Autodesk Inventor part; units mm, degrees
ref_plane "YZ Plane" through (0, 0, 0) normal (1, 0, 0) x (0, 1, 0)
ref_plane "XZ Plane" through (0, 0, 0) normal (0, 1, 0) x (-1, 0, 0)
ref_plane "XY Plane" through (0, 0, 0) normal (0, 0, 1) x (1, 0, 0)
sketch "Sketch1" plane through (0, 0, 0) normal (0, 0, 1) x (1, 0, 0)
  line L0 (-37, 85) -> (37, 85)
  line L1 (37, 85) -> (37, -85)
  line L2 (37, -85) -> (-37, -85)
  line L3 (-37, -85) -> (-37, 85)
  line L4 (-37, 85) -> (37, -85) construction
  line L5 (37, 85) -> (-37, -85) construction
  line L6 (22, 85) -> (-22, 85)
  line L7 (-22, 85) -> (-22, 62)
  line L8 (-22, 62) -> (22, 62)
  line L9 (22, 62) -> (22, 85)
  point P0 (0, 0)
  point P1 (0, 62)
  point P2 (0, 85)
  point P3 (-22, 85)
  dimension "d0" = 74
  dimension "d1" = 170
  dimension "d9" = 44
  dimension "d10" = 23
extrude "Extrusion1" add sketch "Sketch1" along normal blind 5 contours L0 L7 L8 L9 L1 L2 L3
sketch "Sketch2" plane through (0, 0, 0) normal (0, 0, -1) x (-1, 0, 0)
  circle A0 centre (-26, 81) radius 2.5
  line L0 (0, 0) -> (0, 85)
  line L1 (-37, 85) -> (37, 85)
  circle A1 centre (26, 81) radius 2.5
  dimension "d4" = 5
  dimension "d5" = 52
  dimension "d8" = 4
extrude "Extrusion2" cut sketch "Sketch2" against normal blind 4
sketch "Sketch3" plane through (0, 0, 0) normal (0, 0, -1) x (-1, 0, 0)
  line L0 (37, -85) -> (-37, -85)
  line L1 (-37, 85) -> (-37, -85)
  line L2 (-37, -85) -> (37, -85)
  line L3 (37, -85) -> (37, 85)
  line L4 (33, 85) -> (33, -81)
  line L5 (33, -81) -> (-33, -81)
  line L6 (-33, -81) -> (-33, 85)
  line L7 (-37, 85) -> (-22, 85)
  line L8 (-37, 85) -> (-33, 85)
  line L9 (22, 85) -> (37, 85)
  line L10 (33, 85) -> (37, 85)
  line L11 (-33, -81) -> (-27.5, -81)
  line L12 (-27.5, -81) -> (-27.5, -28.7771)
  line L13 (-27.5, -28.7771) -> (-33, -28.7771)
  line L14 (-33, -28.7771) -> (-33, -81)
  line L15 (33, -81) -> (27.5, -81)
  line L16 (27.5, -81) -> (27.5, -28.7771)
  line L17 (27.5, -28.7771) -> (33, -28.7771)
  line L18 (33, -28.7771) -> (33, -81)
  point P0 (0, 0)
  point P1 (33, -28.7771)
  point P2 (-33, -28.7771)
  dimension "d12" = 4
  dimension "d18" = 52.2229
  dimension "d19" = 5.5
  dimension "d20" = 5.5
extrude "Extrusion3" add sketch "Sketch3" along normal blind 22.8316
sketch "Sketch4" plane through (-37, -85, 5) normal (0, -1, 0) x (1, 0, 0)
  line L0 (70, -27.8316) -> (74, -27.8316)
  line L1 (74, -27.8316) -> (0, -27.8316)
  line L2 (0, -27.8316) -> (0, -21.8316)
  line L3 (0, -21.8316) -> (74, -21.8316)
  line L4 (74, -21.8316) -> (74, -27.8316)
  point P0 (37, -5)
  dimension "d15" = 6
  dimension "d21" = 74
extrude "Extrusion4" add sketch "Sketch4" along normal blind 54
chamfer "Chamfer1" distance 10 angle 45 2 edges at (30.25, -28.7771, -22.8316) (-30.25, -28.7771, -22.8316)
sketch "Sketch5" plane through (0, 0, -22.8316) normal (0, 0, -1) x (-1, 0, 0)
  line L0 (-31.85, -29.2771) -> (-31.85, -139.7771)
  line L1 (-31.85, -29.2771) -> (78.65, -29.2771) construction
  circle A0 centre (-31.85, -44.2771) radius 2.5
  circle A1 centre (-31.85, -64.2771) radius 2.5
  circle A2 centre (-31.85, -84.2771) radius 2.5
  circle A3 centre (-31.85, -104.2771) radius 2.5
  circle A4 centre (-31.85, -124.2771) radius 2.5
  line L2 (-27.5, -28.7771) -> (-27.5, -81)
  line L3 (-37, -85) -> (-37, 85)
  line L4 (-27.5, -28.7771) -> (-33, -28.7771)
  line L5 (-37, -139) -> (37, -139)
  line L6 (0, -139) -> (0, -29.2771)
  circle A5 centre (31.85, -44.2771) radius 2.5
  circle A6 centre (31.85, -64.2771) radius 2.5
  circle A7 centre (31.85, -84.2771) radius 2.5
  circle A8 centre (31.85, -104.2771) radius 2.5
  circle A9 centre (31.85, -124.2771) radius 2.5
  point P0 (0, 0)
  point P1 (-31.85, -36)
  dimension "d23" = 110.5
  dimension "d24" = 90
  dimension "d25" = 5
  dimension "d26" = 15
  dimension "d29" = 20
  dimension "d39" = 5.15
  dimension "d40" = 0.5
extrude "Extrusion5" cut sketch "Sketch5" against normal blind 5
fillet "Fillet1" radius 5 4 edges at (37, 0, 5) (-37, 0, 5) (37, -112, -16.8316) (-37, -112, -16.8316)
properties part number "cover^3"
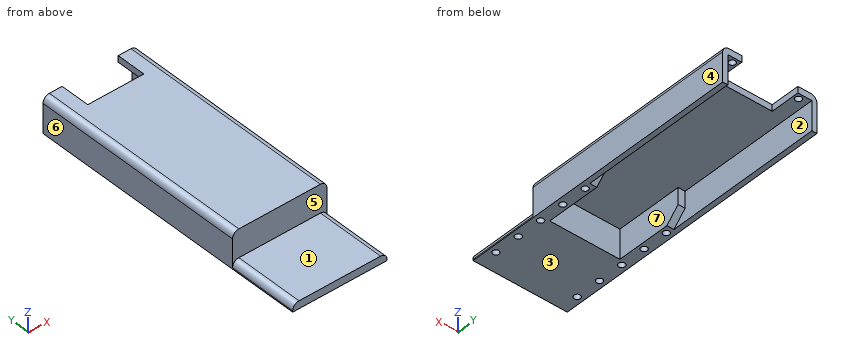
Part model, mm, in its own coordinate system. Face numbers are marked on the shaded views. A direction names the side the tool comes from. Round coordinates to 2 decimals unless told otherwise and drop trailing zeros. Write each loop counter-clockwise with the first axis right and the second up, starting at its lowest first coordinate (ties: lowest second). Pieces come first, ordered by that corner, then holes. Notation, with made-up numbers: (37.25, 44.25) -> (61.25, 44.25) arc R20 ccw to (61.25, 83.25) -> close; hole circle Ø3 at (22.5, -27). An arc over 180 degrees is marked (long way). Return JSON: item names as keys, results as strings. Group by question number.
Q1. Probe L1, parallel to X at y = 70, z = -12.5; L2, parallel to Y at x = 31.85, z = -20.05; L3, parallel to Y at x = 31.85, z = -21.3. List the from-to ranges inside material, lowest first. Write a range as [from, to].
Q2. Pin check, flat tips, straight feed: pin 1 (10 mm diameter, centred on x = -10, y = 2, fed in from -Z); pin 2 (6 mm diameter, centred on x = -10.5, z = -1, fed in from -Y); pin 3 (11.5 mm diameter, centred on x = 9, z = -7.5, fed in from +Y). Stop position of each tip, or through.
Q3. Mould opens along X. For the marked faces 4, 5, 6 and 7 say: pulls with the +X half, pulls with the -X half, needs draft (parallel to the pull), parting line crosses it, or undercut.
Q4. Which spindle directions (+Z, -Z, +X, -X, +Y, -Y) get a long thin tool onto all of the face, cutting with end or side? Do the marked faces 1, 2 and 3. Say none if no direction does.
Q5. Saw through at A-A on y = 81. Write the cut outline in (x, z).
Q6. Saw through at C-C on x = 9. Write the cut outline in (y, z).
Q7. Saw through at B-B on y = 54. Write the cut outline in (x, z).
Answer:
{
 "1": {"L1": "[-37, -33], [33, 37]", "L2": "[-139, -126.78], [-121.78, -106.78], [-101.78, -86.78], [-81.78, -66.78], [-61.78, -46.78], [-41.78, -36]", "L3": "[-139, -126.78], [-121.78, -106.78], [-101.78, -86.78], [-81.78, -66.78], [-61.78, -46.78], [-41.78, -37.25]"},
 "2": {"pin 1": "z = 0", "pin 2": "y = -85", "pin 3": "y = -81"},
 "3": {"face 4": "pulls with the +X half", "face 5": "needs draft", "face 6": "pulls with the -X half", "face 7": "undercut"},
 "4": {"face 1": "+Z, +X, -X, -Y", "face 2": "-Z, +Y", "face 3": "-Z, +X, -X, +Y, -Y"},
 "5": {"outline": "(-37, -22.83) -> (-33, -22.83) -> (-33, 0) -> (-28.5, 0) -> (-28.5, 4) -> (-23.5, 4) -> (-23.5, 0) -> (-22, 0) -> (-22, 5) -> (-32, 5) arc R5 ccw to (-37, 0) -> close; (22, 0) -> (23.5, 0) -> (23.5, 4) -> (28.5, 4) -> (28.5, 0) -> (33, 0) -> (33, -22.83) -> (37, -22.83) -> (37, 0) arc R5 ccw to (32, 5) -> (22, 5) -> close"},
 "6": {"outline": "(-139, -22.83) -> (-81, -22.83) -> (-81, 0) -> (62, 0) -> (62, 5) -> (-85, 5) -> (-85, -16.83) -> (-139, -16.83) -> close"},
 "7": {"outline": "(-37, -22.83) -> (-33, -22.83) -> (-33, 0) -> (33, 0) -> (33, -22.83) -> (37, -22.83) -> (37, 0) arc R5 ccw to (32, 5) -> (-32, 5) arc R5 ccw to (-37, 0) -> close"}
}
